```python
from build123d import *

# Parameters (mm, degrees)
SKETCH1_W           = 300
SKETCH1_H           = 800
SKETCH1_W_2         = 120
SKETCH1_H_2         = 170
BOSS_EXTRUDE1_DEPTH = 1
SKETCH4_R           = 2.5
CUT_EXTRUDE1_DEPTH  = 10
SKETCH5_W           = 12.6
SKETCH5_H           = 19
SKETCH5_W_2         = 12
SKETCH5_H_2         = 12
CUT_EXTRUDE2_DEPTH  = 10


with BuildPart() as part:
    # Sketch1 → Boss-Extrude1 (new body)
    with BuildSketch(Plane.XY):
        Rectangle(SKETCH1_W, SKETCH1_H)
        Rectangle(SKETCH1_W_2, SKETCH1_H_2, mode=Mode.SUBTRACT)
        with Locations((0, 265)):
            Rectangle(SKETCH1_W_2, SKETCH1_H_2, mode=Mode.SUBTRACT)
        with Locations((0, -265)):
            Rectangle(SKETCH1_W_2, SKETCH1_H_2, mode=Mode.SUBTRACT)
    extrude(amount=BOSS_EXTRUDE1_DEPTH)

    # Sketch4 → Cut-Extrude1 (cut)
    with BuildSketch(Plane.XY.offset(1)):
        with Locations((140, 375)):
            Circle(SKETCH4_R)
        with Locations((-140, 375)):
            Circle(SKETCH4_R)
        with Locations((-140, 125)):
            Circle(SKETCH4_R)
        with Locations((-140, -125)):
            Circle(SKETCH4_R)
        with Locations((-140, -375)):
            Circle(SKETCH4_R)
        with Locations((140, 125)):
            Circle(SKETCH4_R)
        with Locations((140, -125)):
            Circle(SKETCH4_R)
        with Locations((140, -375)):
            Circle(SKETCH4_R)
    extrude(amount=-CUT_EXTRUDE1_DEPTH, mode=Mode.SUBTRACT)

    # Sketch5 → Cut-Extrude2 (cut)
    with BuildSketch(Plane.XY.offset(1)):
        with Locations((-113.7, 189.5)):
            Rectangle(SKETCH5_W, SKETCH5_H)
        with Locations((-113.7, -75.5)):
            Rectangle(SKETCH5_W, SKETCH5_H)
        with Locations((-113.7, -340.5)):
            Rectangle(SKETCH5_W, SKETCH5_H)
        with Locations((-114, -20)):
            Rectangle(SKETCH5_W_2, SKETCH5_H_2)
        with Locations((-114, 245)):
            Rectangle(SKETCH5_W_2, SKETCH5_H_2)
        with Locations((-114, -285)):
            Rectangle(SKETCH5_W_2, SKETCH5_H_2)
    extrude(amount=-CUT_EXTRUDE2_DEPTH, mode=Mode.SUBTRACT)


solid = part.part
```
CAD build for the part. Positions are in the model's coordinates, mm. Coordinates: 2 decimals unless noted, no trailing zeros. Loops run counter-clockwise (first coordinate to the right, second up) from the corner with the lowest first, then second, coordinate; pieces in that order, holes last. Notation, with made-up numbers: (-27, -34.75) - (-13, -34.75) arc R25 cw to (-13, -1.75) - close; hole circle Ø10 at (1.5, 52.5). An arc over 180 degrees is marked (long way). Return JSON: item names as keys, results as strings.
1. Drop a flat-ended pin along its axis: pin 1 (4 mm diameter, centred on x = 140, y = -125, fed in from +Z) (3 decimals). Give the stop position or say it passes through.
Result:
{"pin 1": "passes through"}
2. Band-saw the part on C-C (z = 0.8). State how many separate pieces and enclosed holes the cut face has, and give its area (3 significant figures).
Result:
{"separate pieces": "1", "enclosed holes": "17", "area": "177,000 mm2"}
3. Band-saw the part on B-B (y = 27). Give the cut face in (x, z).
Result:
{"outline": "(-150, 0) - (-60, 0) - (-60, 1) - (-150, 1) - close; (60, 0) - (150, 0) - (150, 1) - (60, 1) - close"}
4. Probe L1, parallel to Y at x = -8.5, z = 0.65; L2, parallel to Y at x = -140, z = 0.75; L3, parallel to X at y = 375, z = 0.8. List the from-to ranges inside material, lowest first. Write a range as from..to.
Result:
{"L1": "y = -400..-350, -180..-85, 85..180, 350..400", "L2": "y = -400..-377.5, -372.5..-127.5, -122.5..122.5, 127.5..372.5, 377.5..400", "L3": "x = -150..-142.5, -137.5..137.5, 142.5..150"}
5. Band-saw the part on A-A (x = 17). Give the cut face in (y, z).
Result:
{"outline": "(-400, 0) - (-350, 0) - (-350, 1) - (-400, 1) - close; (-180, 0) - (-85, 0) - (-85, 1) - (-180, 1) - close; (85, 0) - (180, 0) - (180, 1) - (85, 1) - close; (350, 0) - (400, 0) - (400, 1) - (350, 1) - close"}
